For this review, use the dimensioned drawing (mm, ordinates from the lowest corner) and the shaded views. Coordinates: 2 decimals unless noted, no trailing zeros. Order: outer loops, then holes, each group sorted by start corner. A loop starts at its lowest first (then second) coordinate and runs counter-clockwise, first axis right, second up. Notation, with made-up numbers: (34.5, -6) -> (83.5, -6) arc R27 ccw to (83.5, 24) -> close; hole circle Ø3 at (48.5, 37.25). An arc over 180 degrees is marked (long way). Use CSV: the item, a comma, the result in double quotes. Start each with the question number.
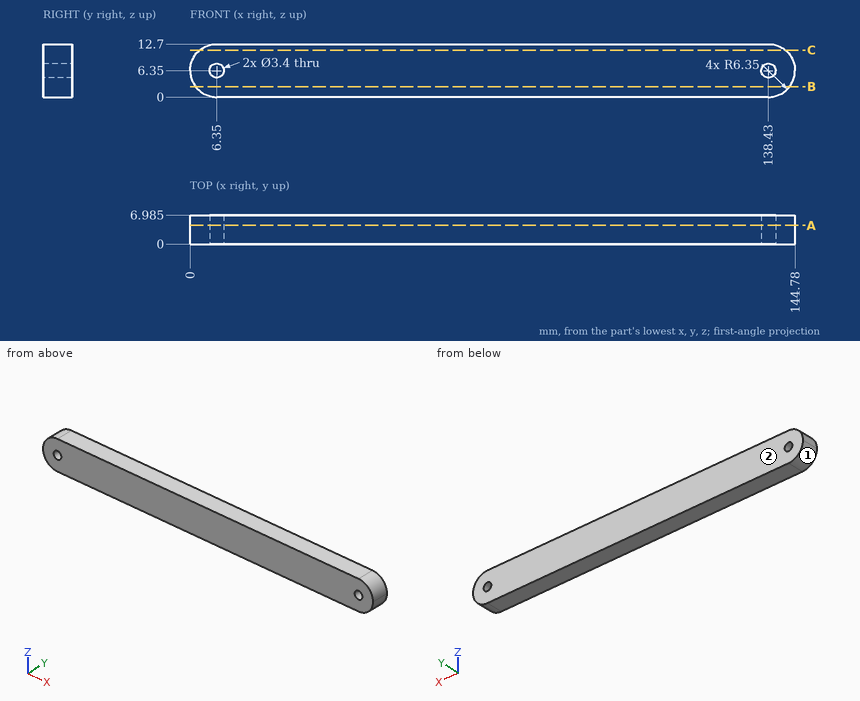
Q1. Draft analysis for pull direction X (two halves, no side actions). For the marked faces 1 and 2, state which applies: +X half, -X half, draft (parallel to the pull), parting line (faces both ways), or undercut.
Q2. Add section A-A, the plane y = 4.5. State how many separate pieces and enclosed holes the cut face has, then the cut area to 3 significant figures.
Q3. Add section B-B, the plane z = 2.5. State the section outline as (x, y) points (3 decimals).
Q4. To check wall thickness, follow probe 1 along X at (y, z) = (3.25, 6.35); probe 2 along Z at (x, y) = (6.35, 5.25); probe 3 along X at (y, z) = (5.5, 5.5). State the ranges of each line that lie inside material, in increasing order.
Q5. Add section C-C, the plane z = 11.25. State the section outline as (x, y) points (3 decimals), then the cut area to 3 significant figures.
Answer block:
1,face 1,"-X half"
1,face 2,"draft"
2,separate pieces,"1"
2,enclosed holes,"2"
2,area,"1,790 mm²"
3,outline,"(1.3, 0) -> (143.48, 0) -> (143.48, 6.985) -> (1.3, 6.985) -> close"
4,probe 1,"x = 0 to 4.65, 8.05 to 136.73, 140.13 to 144.78"
4,probe 2,"z = 0 to 4.65, 8.05 to 12.7"
4,probe 3,"x = 0.06 to 4.88, 7.82 to 136.96, 139.9 to 144.72"
5,outline,"(2.311, 0) -> (142.469, 0) -> (142.469, 6.985) -> (2.311, 6.985) -> close"
5,area,"979 mm²"
